from build123d import *

# Parameters (mm, degrees)
SKETCH1_R           = 19
SKETCH1_R_2         = 3
BOSS_EXTRUDE1_DEPTH = 3
SKETCH2_R           = 4
BOSS_EXTRUDE2_DEPTH = 16
CUT_EXTRUDE1_START  = -6
CUT_EXTRUDE1_DEPTH  = 6
BOSS_EXTRUDE3_START = 3
SKETCH5_R           = 19
SKETCH5_R_2         = 1.6
BOSS_EXTRUDE3_DEPTH = 3


with BuildPart() as part:
    # Sketch1 → Boss-Extrude1 (new body)
    with BuildSketch(Plane(origin=(0, 0, 0), x_dir=(1, 0, 0), z_dir=(0, 1, 0))):
        with Locations(Location((0, 0, 0), (0, 0, 270))):
            Circle(SKETCH1_R)
        with Locations(Location((0, 15.5, 0), (0, 0, 270))):
            Circle(SKETCH1_R_2, mode=Mode.SUBTRACT)
        with Locations(Location((15.5, 0, 0), (0, 0, 270))):
            Circle(SKETCH1_R_2, mode=Mode.SUBTRACT)
        with Locations(Location((0, -15.5, 0), (0, 0, 270))):
            Circle(SKETCH1_R_2, mode=Mode.SUBTRACT)
        with Locations(Location((-15.5, 0, 0), (0, 0, 270))):
            Circle(SKETCH1_R_2, mode=Mode.SUBTRACT)
    extrude(amount=BOSS_EXTRUDE1_DEPTH)

    # Sketch2 → Boss-Extrude2 (add)
    with BuildSketch(Plane(origin=(0, 3, 0), x_dir=(1, 0, 0), z_dir=(0, 1, 0))):
        with Locations(Location((0, 0, 0), (0, 0, 270))):
            Circle(SKETCH2_R)
    extrude(amount=BOSS_EXTRUDE2_DEPTH)

    # Sketch4 → Cut-Extrude1 (cut)
    with BuildSketch(Plane(origin=(0, 19, 0), x_dir=(1, 0, 0), z_dir=(0, 1, 0)).offset(CUT_EXTRUDE1_START)):
        with BuildLine():
            Line((-2.5, -3.122498999), (2.5, -3.122498999))
            ThreePointArc((2.5, -3.122498999), (0, -4), (-2.5, -3.122498999))
        make_face()
        with BuildLine():
            Line((3.122498999, 2.5), (3.122498999, -2.5))
            ThreePointArc((3.122498999, -2.5), (4, 0), (3.122498999, 2.5))
        make_face()
    extrude(amount=CUT_EXTRUDE1_DEPTH, mode=Mode.SUBTRACT)

    # Sketch5 → Boss-Extrude3 (add)
    with BuildSketch(Plane.XZ.offset(BOSS_EXTRUDE3_START)):
        with Locations(Location((0, 0, 0), (0, 0, 270))):
            Circle(SKETCH5_R)
        with Locations(Location((0, 15.5, 0), (0, 0, 270))):
            Circle(SKETCH5_R_2, mode=Mode.SUBTRACT)
        with Locations(Location((-15.5, 0, 0), (0, 0, 270))):
            Circle(SKETCH5_R_2, mode=Mode.SUBTRACT)
        with Locations(Location((0, -15.5, 0), (0, 0, 270))):
            Circle(SKETCH5_R_2, mode=Mode.SUBTRACT)
        with Locations(Location((15.5, 0, 0), (0, 0, 270))):
            Circle(SKETCH5_R_2, mode=Mode.SUBTRACT)
    extrude(amount=-BOSS_EXTRUDE3_DEPTH)


solid = part.part
Here's how the part is built. I have some questions about the finished solid (model axes, mm). A direction names the side the tool comes from. Give positions to 0.01 mm unless a question says otherwise; leave off trailing zeros. Order: outer loops, then holes, each group sorted by start corner. A loop starts at its lowest first (then second) coordinate and runs counter-clockwise, first axis right, second up. Notation, with made-up numbers: (-19.75, 22.25) -> (10.25, 22.25) arc R19 cw to (10.25, 42.25) -> close; hole circle Ø7 at (55, -31). An arc over 180 degrees is marked (long way). One line per item, written item: value. Start each with the question number.
1. For faces 1 (the face through (0, 16, 3.122)), 2 (the face through (0.07, -1.52, -13.9)), 3 (the face through (3.5, 13, 0)), 4 (the face through (0.1, 1.5, -18.5)), which set-ups out of +Z, -Z, +X, -X, +Y, -Y let a thin tool reach every point of the face, with its end or its side?
2. Will these pins go through, and if not, where does the flat tip stop? pin 1 Ø8 at (y, z) = (0.5, -10) entering from +X; pin 2 Ø8 at (x, z) = (0, 15.5) entering from +Y; pin 3 Ø5.5 at (y, z) = (17, 0) entering from +X.
3. Imagine slicing it at A-A, the plane x = 0. List the corners of the cut face in (y, z) for me, plus the area to 3 significant figures.
4. Imagine slicing it at C-C, the plane y = 2.5. List the corners of the cut face in (x, z) for me, plus the area to 3 significant figures.
5. Imagine slicing it at D-D, the plane z = 15.5. List the corners of the cut face in (x, y) for me, plus the area to 3 significant figures.
6. I need wall thicknesses on probe 1 along X at (y, z) = (-1.6, 0); probe 2 along Y at (x, z) = (-9, 2); probe 3 along X at (y, z) = (-0.7, 15.5). Which ranges of each line are inside material? Lowest first, please. Write a range as from..to.
7. We'd pull the mould along Z, two halves only. Please class faces 5 (the face through (0, -3, 0)), 6 (the face through (17.086, -1.521, 0.208)), 7 (the face through (-2.4, 9.1, -3.2)): released by +Z, released by -Z, zero draft, split by the parting line, or undercut.
8. Imagine slicing it at B-B, the plane z = 0. List the corners of the cut face in (x, y) for me, plus the area to 3 significant figures.
Values follow:
1. face 1: +Z, +X, -X, +Y
1. face 2: +Y, -Y
1. face 3: +Z, -Z, +X, +Y
1. face 4: +Y
2. pin 1: stops at x = 18.03
2. pin 2: stops at y = 3
2. pin 3: stops at x = 3.12
3. outline: (-3, -19) -> (3, -19) -> (3, -18.5) -> (0, -18.5) -> (0, -17.1) -> (-3, -17.1) -> close; (-3, -13.9) -> (0, -13.9) -> (0, -12.5) -> (3, -12.5) -> (3, -4) -> (19, -4) -> (19, 3.12) -> (13, 3.12) -> (13, 4) -> (3, 4) -> (3, 12.5) -> (0, 12.5) -> (0, 13.9) -> (-3, 13.9) -> close; (-3, 17.1) -> (0, 17.1) -> (0, 18.5) -> (3, 18.5) -> (3, 19) -> (-3, 19) -> close
3. area: 296 mm2
4. outline: circle Ø38 at (0, 0); hole circle Ø6 at (-15.5, 0); hole circle Ø6 at (0, -15.5); hole circle Ø6 at (0, 15.5); hole circle Ø6 at (15.5, 0)
4. area: 1,020 mm2
5. outline: (-10.99, -3) -> (-1.6, -3) -> (-1.6, 0) -> (-3, 0) -> (-3, 3) -> (-10.99, 3) -> close; (1.6, -3) -> (10.99, -3) -> (10.99, 3) -> (3, 3) -> (3, 0) -> (1.6, 0) -> close
5. area: 104 mm2
6. probe 1: x = -19..-17.1, -13.9..13.9, 17.1..19
6. probe 2: y = -3..3
6. probe 3: x = -10.99..-1.6, 1.6..10.99
7. face 5: zero draft
7. face 6: undercut
7. face 7: split by the parting line
8. outline: (-19, -3) -> (-17.1, -3) -> (-17.1, 0) -> (-18.5, 0) -> (-18.5, 3) -> (-19, 3) -> close; (-13.9, -3) -> (13.9, -3) -> (13.9, 0) -> (12.5, 0) -> (12.5, 3) -> (4, 3) -> (4, 13) -> (3.12, 13) -> (3.12, 19) -> (-4, 19) -> (-4, 3) -> (-12.5, 3) -> (-12.5, 0) -> (-13.9, 0) -> close; (17.1, -3) -> (19, -3) -> (19, 3) -> (18.5, 3) -> (18.5, 0) -> (17.1, 0) -> close
8. area: 296 mm2
